Answer from the drawing. Dimensions are ordinates in mm from the lowest x, y and z of the part. A direction names the side the tool comes from. Coordinates: 2 decimals unless noted, no trailing zeros. Write each loop counter-clockwise with the first axis right and the second up, starting at its lowest first coordinate (ties: lowest second). Pieces come first, ordered by that corner, then holes.
1) The part is cut by section C-C (y = 42.5). Determine the outline of the cut face in (x, z) (1 decimal), then the cut area to 3 significant figures.
2) The part is cut by section A-A (x = 16). Determine the outline of the cut face in (y, z).
3) Each of these flat-tipped pins is pushed along its axis until it touches: pin 1 Ø12 at (y, z) = (26, 13) entering from -X; pin 2 Ø2 at (x, y) = (43, 2.5) entering from +Z. Where does it stop, or does it pass through?
4) Which of the six approach directions +Z, -Z, +X, -X, +Y, -Y give full straight-line access (tool end or side, diameter ignored) to the marked faces 1 and 2?
5) Determine the mould class of the marked faces 3, 4, 5 and 6 for opening direction Y: +Y half, -Y half, draft (parallel to the pull), parting line (faces both ways), or undercut.
6) The part is cut by section B-B (z = 6). Determine the outline of the cut face in (x, y) (1 decimal), then the cut area to 3 significant figures.
7) Find the intervals of material crossed by line 1 (Y direction, x = 78, z = 32); line 2 (X direction, y = 11.5, z = 33) (1 decimal); line 3 (X direction, y = 4, z = 35), in increasing order.
8) The part is cut by section D-D (y = 23). Determine the outline of the cut face in (x, z) (1 decimal).
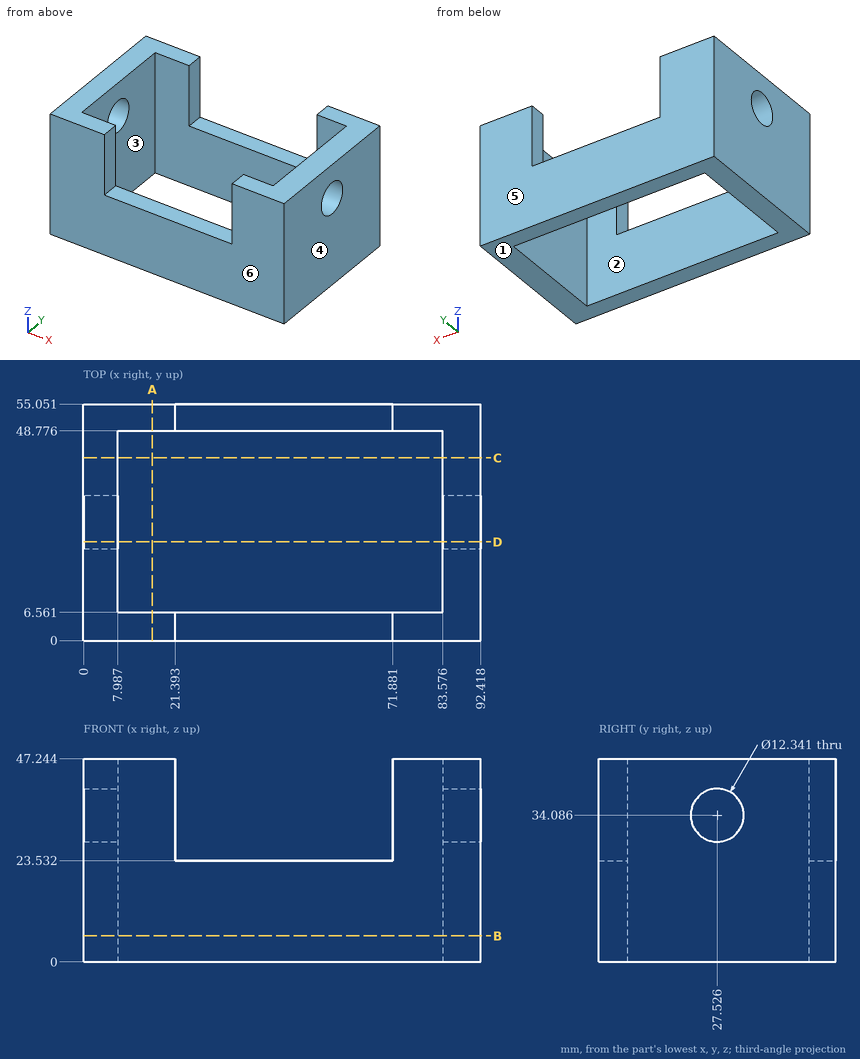
Reported:
1. outline: (0, 0) - (8, 0) - (8, 47.2) - (0, 47.2) - close; (83.6, 0) - (92.4, 0) - (92.4, 47.2) - (83.6, 47.2) - close
1. area: 795 mm2
2. outline: (0, 0) - (6.56, 0) - (6.56, 47.24) - (0, 47.24) - close; (48.78, 0) - (55.05, 0) - (55.05, 47.24) - (48.78, 47.24) - close
3. pin 1: stops at x = 0
3. pin 2: stops at z = 23.53
4. face 1: -Z, +X, -X, +Y, -Y
4. face 2: +Z, -Z
5. face 3: undercut
5. face 4: draft
5. face 5: +Y half
5. face 6: -Y half
6. outline: (0, 0) - (92.4, 0) - (92.4, 55.1) - (0, 55.1) - close; hole (8, 6.6) - (83.6, 6.6) - (83.6, 48.8) - (8, 48.8) - close
6. area: 1,900 mm2
7. line 1: y = 0 to 6.56, 48.78 to 55.05
7. line 2: x = 0 to 8, 83.6 to 92.4
7. line 3: x = 0 to 21.39, 71.88 to 92.42
8. outline: (0, 0) - (8, 0) - (8, 29.9) - (0, 29.9) - close; (0, 38.3) - (8, 38.3) - (8, 47.2) - (0, 47.2) - close; (83.6, 0) - (92.4, 0) - (92.4, 29.9) - (83.6, 29.9) - close; (83.6, 38.3) - (92.4, 38.3) - (92.4, 47.2) - (83.6, 47.2) - close
